Verification items for the finished model (mm, model axes). Face numbers are marked on the shaded views. Coordinates: 2 decimals unless noted, no trailing zeros. Write each loop counter-clockwise with the first axis right and the second up, starting at its lowest first coordinate (ties: lowest second). Pieces come first, ordered by that corner, then holes. Notation, with made-up numbers: (-13, -20) -> (-2, -20) arc R18 cw to (-2, -2) -> close; hole circle Ø10 at (32, 55). An arc over 180 degrees is marked (long way). Answer in a Markdown table with one row per item.
```python
from build123d import *

# Parameters (mm, degrees)
F0_W     = 7.62
F0_H     = 5.08
F1_DEPTH = 25.4


with BuildPart() as f1:
    # F0 (on Top) → F1 (new body)
    with BuildSketch(Plane.XY):
        with BuildLine():
            ThreePointArc((63.5, -50.8), (81.460512, -43.360512), (88.9, -25.4))
            Line((88.9, -25.4), (88.9, 25.4))
            ThreePointArc((88.9, 25.4), (81.460512, 43.360512), (63.5, 50.8))
            ThreePointArc((63.5, 50.8), (0, 46.582226), (-63.5, 50.8))
            ThreePointArc((-63.5, 50.8), (-81.460512, 43.360512), (-88.9, 25.4))
            Line((-88.9, 25.4), (-88.9, -25.4))
            ThreePointArc((-88.9, -25.4), (-81.460512, -43.360512), (-63.5, -50.8))
            ThreePointArc((-63.5, -50.8), (0, -46.582226), (63.5, -50.8))
        make_face()
        with Locations((-54.61, -33.02)):
            Rectangle(F0_W, F0_H, mode=Mode.SUBTRACT)
        with Locations((54.61, -33.02)):
            Rectangle(F0_W, F0_H, mode=Mode.SUBTRACT)
        with Locations((-54.61, 33.02)):
            Rectangle(F0_W, F0_H, mode=Mode.SUBTRACT)
        with Locations((54.61, 33.02)):
            Rectangle(F0_W, F0_H, mode=Mode.SUBTRACT)
    extrude(amount=F1_DEPTH)


solid = f1.part
```
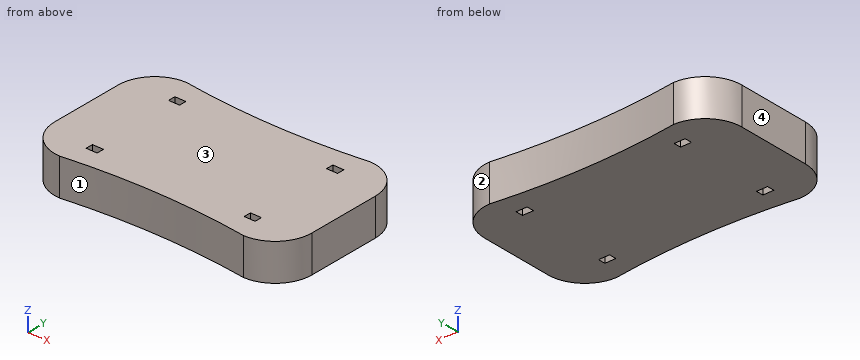
1. Sectioned sample at D-D, the plane x = 4. Record the cut outline in (y, z).
Findings below:
| item | result |
|---|---|
| outline | (-46.6, 0) -> (46.6, 0) -> (46.6, 25.4) -> (-46.6, 25.4) -> close |
2. Go/stop test with flat-tipped pins: pin 1 (3 mm diameter, centred on x = 56.5, z = 4, fed in from +Y); pin 2 (5.5 mm diameter, centred on y = 33, z = 6.5, fed in from -X); pin 3 (6 mm diameter, centred on x = -24, z = 10, fed in from -Y). Record where each tip stops, or that it passes through.
Findings below:
| item | result |
|---|---|
| pin 1 | stops at y = 50.1 |
| pin 2 | stops at x = -88.43 |
| pin 3 | stops at y = -47.34 |
3. Release check for a two-part mould opening along X. For the marked faces 1, 2, 3 and 4 record: released by +X, released by -X, zero draft, split by the parting line, or undercut.
Findings below:
| item | result |
|---|---|
| face 1 | undercut |
| face 2 | released by +X |
| face 3 | zero draft |
| face 4 | released by -X |
4. Sectioned sample at C-C, the plane y = 43. Record the cut outline in (x, z), and give its area (3 significant figures).
Findings below:
| item | result |
|---|---|
| outline | (-81.81, 0) -> (81.81, 0) -> (81.81, 25.4) -> (-81.81, 25.4) -> close |
| area | 4,160 mm² |
5. Material ranges on probe 1 along X at (y, z) = (34, 5.5); probe 2 along X at (y, z) = (31, 19.25); probe 3 along Y at (x, z) = (45.5, 3.5), recorded low to high. Write a range as from..to.
Findings below:
| item | result |
|---|---|
| probe 1 | x = -87.4..-58.42, -50.8..50.8, 58.42..87.4 |
| probe 2 | x = -88.27..-58.42, -50.8..50.8, 58.42..88.27 |
| probe 3 | y = -48.74..48.74 |
6. Sectioned sample at B-B, the plane x = 53.5. Record the cut outline in (y, z), and give its area (3 significant figures).
Findings below:
| item | result |
|---|---|
| outline | (-49.57, 0) -> (-35.56, 0) -> (-35.56, 25.4) -> (-49.57, 25.4) -> close; (-30.48, 0) -> (30.48, 0) -> (30.48, 25.4) -> (-30.48, 25.4) -> close; (35.56, 0) -> (49.57, 0) -> (49.57, 25.4) -> (35.56, 25.4) -> close |
| area | 2,260 mm² |
7. Sectioned sample at A-A, the plane z = 11. Record the cut outline in (x, y).
Findings below:
| item | result |
|---|---|
| outline | (-88.9, -25.4) arc R25.4 ccw to (-63.5, -50.8) arc R480.12 cw to (63.5, -50.8) arc R25.4 ccw to (88.9, -25.4) -> (88.9, 25.4) arc R25.4 ccw to (63.5, 50.8) arc R480.12 cw to (-63.5, 50.8) arc R25.4 ccw to (-88.9, 25.4) -> close; hole (-58.42, -35.56) -> (-50.8, -35.56) -> (-50.8, -30.48) -> (-58.42, -30.48) -> close; hole (-58.42, 30.48) -> (-50.8, 30.48) -> (-50.8, 35.56) -> (-58.42, 35.56) -> close; hole (50.8, -35.56) -> (58.42, -35.56) -> (58.42, -30.48) -> (50.8, -30.48) -> close; hole (50.8, 30.48) -> (58.42, 30.48) -> (58.42, 35.56) -> (50.8, 35.56) -> close |
